from build123d import *

# Parameters (mm, degrees)
SKETCH1_W           = 180
SKETCH1_H           = 205
BOSS_EXTRUDE1_DEPTH = 10
SKETCH2_W           = 5
SKETCH2_H           = 180
BOSS_EXTRUDE2_DEPTH = 5
SKETCH5_W           = 21
SKETCH5_H           = 3.5
CUT_EXTRUDE3_DEPTH  = 10
SKETCH6_W           = 20.5
SKETCH6_H           = 3.2
CUT_EXTRUDE4_DEPTH  = 10


with BuildPart() as part:
    # Sketch1 → Boss-Extrude1 (new body)
    with BuildSketch(Plane(origin=(0, 0, 0), x_dir=(0, 1, 0), z_dir=(0, 0, 1))):
        Rectangle(SKETCH1_W, SKETCH1_H)
    extrude(amount=BOSS_EXTRUDE1_DEPTH)

    # Sketch2 → Boss-Extrude2 (add)
    with BuildSketch(Plane.XY.offset(10)):
        with Locations((100, 0)):
            Rectangle(SKETCH2_W, SKETCH2_H)
    extrude(amount=BOSS_EXTRUDE2_DEPTH)

    # Sketch5 → Cut-Extrude3 (cut)
    with BuildSketch(Plane(origin=(-102.5, 0, 0), x_dir=(0, -1, 0), z_dir=(-1, 0, 0))):
        with Locations((-40.5, 5)):
            Rectangle(SKETCH5_W, SKETCH5_H)
        with Locations((40.5, 5)):
            Rectangle(SKETCH5_W, SKETCH5_H)
    extrude(amount=-CUT_EXTRUDE3_DEPTH, mode=Mode.SUBTRACT)

    # Sketch6 → Cut-Extrude4 (cut)
    with BuildSketch(Plane.XZ.offset(90)):
        with Locations((70, 5)):
            Rectangle(SKETCH6_W, SKETCH6_H)
        with Locations((-70, 5)):
            Rectangle(SKETCH6_W, SKETCH6_H)
    cut_extrude4 = extrude(amount=-CUT_EXTRUDE4_DEPTH, mode=Mode.SUBTRACT)

    # Mirror1: Cut-Extrude4 across plane
    add(cut_extrude4.mirror(Plane.ZX), mode=Mode.SUBTRACT)


solid = part.part
Can you work these out from the model? Positions are in its coordinate system, mm. A direction names the side the tool comes from. Give positions to 0.01 mm unless a question says otherwise; leave off trailing zeros. Loops run counter-clockwise (first coordinate to the right, second up) from the corner with the lowest first, then second, coordinate; pieces in that order, holes last. Notation, with made-up numbers: (73, -37) -> (121, -37) arc R33 cw to (121, -2) -> close; hole circle Ø5 at (63.25, 84.25). An arc over 180 degrees is marked (long way). Write item = value, one per line.
1) For faces 1 (the flat face through (70, 85, 6.6)), 2 (the flat face through (-98, 41, 6.75)), 3 (the flat face through (70, -85, 3.4)), which set-ups out of +Z, -Z, +X, -X, +Y, -Y let a thin tool reach every point of the face, with its end or its side?
Check result:
face_1 = +Y
face_2 = -X
face_3 = -Y
2) Thinking about a two-plate mould opening in X: for faces 4 (the flat face through (-70, -85, 6.6)), 5 (the flat face through (102.5, -1, 7)), 6 (the flat face through (-98, 41, 3.25)), which applies, released by +X, released by -X, zero draft, split by the parting line, or undercut?
Check result:
face_4 = undercut
face_5 = released by +X
face_6 = zero draft
3) Suppose I cut it at A-A on y = -33. Write out the boundary of the cut face in (x, z).
Check result:
outline = (-102.5, 0) -> (102.5, 0) -> (102.5, 15) -> (97.5, 15) -> (97.5, 10) -> (-102.5, 10) -> (-102.5, 6.75) -> (-92.5, 6.75) -> (-92.5, 3.25) -> (-102.5, 3.25) -> close
4) Suppose I cut it at B-B on x = 12. Write out the boundary of the cut face in (y, z), then the cut area to 3 significant figures.
Check result:
outline = (-90, 0) -> (90, 0) -> (90, 10) -> (-90, 10) -> close
area = 1,800 mm2
5) I need wall thicknesses on L1, parallel to Z at x = -19.5, y = -47.5; L2, parallel to Y at x = -62, z = 5; L3, parallel to X at y = 15.5, z = 13.75. Which ranges of each line are inside material? Lowest first, please. Write a range as from..to.
Check result:
L1 = 0..10
L2 = -80..80
L3 = 97.5..102.5
6) Will these pins go through, and if not, where does the flat tip stop? pin 1 (3.5 mm diameter, centred on x = 70, z = 5, fed in from +Y); pin 2 (1 mm diameter, centred on x = 69, z = 5.5, fed in from -Y); pin 3 (2 mm diameter, centred on x = 16.5, z = 12.5, fed in from +Y); pin 4 (2 mm diameter, centred on y = 22.5, z = 11.5, fed in from -X).
Check result:
pin_1 = 90
pin_2 = -80
pin_3 = through
pin_4 = 97.5
